Model file for the job. Use its own axes, mm. Face numbers are marked on the shaded views. A direction names the side the tool comes from. Give positions to 0.01 mm unless a question says otherwise; leave off trailing zeros. Loops run counter-clockwise (first coordinate to the right, second up) from the corner with the lowest first, then second, coordinate; pieces in that order, holes last. Notation, with made-up numbers: (79.25, 20) -> (128.25, 20) arc R24 cw to (128.25, 38) -> close; hole circle Ø6 at (54.5, -12.5). An arc over 180 degrees is marked (long way). Use CSV: the item, a comma, the result in double quotes. Start each with the question number.
(1) Cut at D-D on x = 444.5. Write the cut outline in (y, z), then the cut area to 3 significant figures.
(2) 3-axis set-ups, long thin cutter, end or side, ignore diameter. For the marked faces 5, 6 and 7: which of +Z, -Z, +X, -X, +Y, -Y reach the whole face in a straight line?
(3) Cut at C-C on z = 6. Write the cut outline in (x, y) (3 decimals).
(4) Pull direction Z, two halves, no side cores. Call the marked faces 1, 2, 3 and 4: pulls with the +Z half, pulls with the -Z half, needs draft (parallel to the pull), parting line crosses it, or undercut.
(5) Cut at A-A on y = 120.5. Write the cut outline in (x, z).
(6) Drill centre lines: probe 1 along Y at (x, z) = (442, -6.5); probe 2 along Z at (x, y) = (450.5, 118); probe 3 along X at (y, z) = (130, 14). Where is each one in solid material? Low to high.
(7) Flat gauge pins, fed straight in: pin 1 (10.5 mm diameter, centred on x = 440.5, y = 127, fed in from -Z); pin 2 (6.5 mm diameter, centred on x = 445.5, y = 125, fed in from +Z); pin 3 (8 mm diameter, centred on x = 445.5, z = -11.5, fed in from +Y). Where does each tip first touch, or does it go through?
(8) Cut at B-B on x = 436.5. Write the cut outline in (y, z), then the cut area to 3 significant figures.
from build123d import *

# Parameters (mm, degrees)
SKETCH1_R           = 3.175
BOSS_EXTRUDE1_DEPTH = 22.098
SKETCH2_R           = 3.175
BOSS_EXTRUDE2_DEPTH = 5.588


with BuildPart() as part:
    # Sketch1 → Boss-Extrude1 (new body)
    with BuildSketch(Plane.XY):
        Polygon((430.481837091, 135.188251435), (451.546293611, 135.188251435), (451.139125986, 110.702070678), (430.481837091, 110.702070678), align=None)
        with Locations(Location((437.331098026, 130.5, 0), (0, 0, 180))):
            Circle(SKETCH1_R, mode=Mode.SUBTRACT)
        with Locations(Location((437.164813366, 120.5, 0), (0, 0, 180))):
            Circle(SKETCH1_R, mode=Mode.SUBTRACT)
    extrude(amount=BOSS_EXTRUDE1_DEPTH)

    # Sketch2 → Boss-Extrude2 (add)
    with BuildSketch(Plane(origin=(0, 110.702070678, 0), x_dir=(1, 0, 0), z_dir=(0, 1, 0))):
        Polygon((431.295573302, -44.662968175), (440.840064565, 23.249615979), (462.21995217, 20.24486873), (452.675460906, -47.667715425), align=None)
        with Locations(Location((443.222765971, -37.361858669, 0), (0, 0, 270))):
            Circle(SKETCH2_R, mode=Mode.SUBTRACT)
        with Locations(Location((450.2927595, 12.943759223, 0), (0, 0, 270))):
            Circle(SKETCH2_R, mode=Mode.SUBTRACT)
    extrude(amount=-BOSS_EXTRUDE2_DEPTH)


solid = part.part
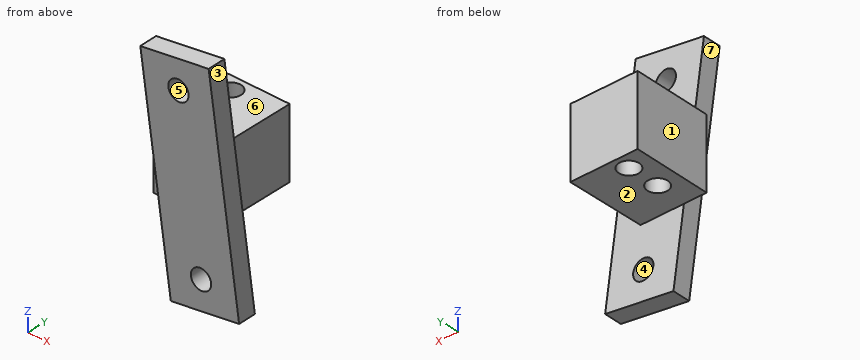
Check result:
1,outline,"(105.11, -22.74) -> (110.7, -22.74) -> (110.7, 0) -> (135.19, 0) -> (135.19, 22.1) -> (110.7, 22.1) -> (110.7, 34.46) -> (105.11, 34.46) -> close; (105.11, 40.27) -> (110.7, 40.27) -> (110.7, 46.52) -> (105.11, 46.52) -> close"
1,area,"896 mm²"
2,face 5,"+Y, -Y"
2,face 6,"+Z, +X, -X, +Y"
2,face 7,"-Z, -X, -Y"
3,outline,"(430.482, 110.702) -> (436.729, 110.702) -> (436.729, 105.114) -> (458.531, 105.114) -> (458.531, 110.702) -> (451.139, 110.702) -> (451.546, 135.188) -> (430.482, 135.188) -> close; hole circle Ø6.35 at (437.165, 120.5); hole circle Ø6.35 at (437.331, 130.5)"
4,face 1,"needs draft"
4,face 2,"pulls with the -Z half"
4,face 3,"pulls with the +Z half"
4,face 4,"undercut"
5,outline,"(430.48, 0) -> (433.99, 0) -> (433.99, 22.1) -> (430.48, 22.1) -> close; (440.34, 0) -> (451.3, 0) -> (451.3, 22.1) -> (440.34, 22.1) -> close"
6,probe 1,"105.11 to 110.7"
6,probe 2,"0 to 22.1"
6,probe 3,"430.48 to 434.2, 440.47 to 451.46"
7,pin 1,"z = 0"
7,pin 2,"z = 22.1"
7,pin 3,"y = 110.7"
8,outline,"(105.11, 7.63) -> (110.7, 7.63) -> (110.7, 0) -> (117.4, 0) -> (117.4, 22.1) -> (110.7, 22.1) -> (110.7, 45.39) -> (105.11, 45.39) -> close; (123.6, 0) -> (127.44, 0) -> (127.44, 22.1) -> (123.6, 22.1) -> close; (133.56, 0) -> (135.19, 0) -> (135.19, 22.1) -> (133.56, 22.1) -> close"
8,area,"479 mm²"
